Source: CAD feature listing. Evaluate the final solid. Frame: model axes, mm. A direction names the side the tool comes from. Round coordinates to 2 decimals unless told otherwise and drop trailing zeros. Order: outer loops, then holes, each group sorted by start corner. A loop starts at its lowest first (then second) coordinate and runs counter-clockwise, first axis right, second up. Notation, with made-up numbers: (11.5, 50.25) -> (47.5, 50.25) arc R29 ccw to (47.5, 85.25) -> close; hole circle Ø7 at (-26, 66). An arc over 180 degrees is marked (long way). Write item = value, one per line. Start each with the question number.
(1) Cut plane D-D on x = -1.5. Return the cut outline in (y, z), then the cut area to 3 significant figures.
(2) Draft query along Y for faces 1 (the face through (0, 11.43, 11)), 2 (the face through (0, 1, 5)), 3 (the face through (2.57, 8.7, 11.45)), 4 (the face through (-2, 0, 8)). Return one class per face: released by +Y, released by -Y, zero draft, split by the parting line, or undercut.
(3) Ray query, line 1 (X direction, y = 2, z = 5); line 2 (Z direction, x = 7.5, y = 4.25); line 3 (Z direction, x = -6.25, y = 1.5). Return the intervals inside material, ascending.
(4) Reachability of faces 5 (the face through (-5, 1, 0)), 6 (the face through (-7.5, 2.54, 5)) from +Z, -Z, +X, -X, +Y, -Y: full face, straight path, thin tool, end or side. Return the list, or none.
(5) Cut plane C-C on x = -6.25. Return the cut outline in (y, z).
(6) Cut plane B-B on z = 5.08. Return the cut outline in (x, y) (3 decimals).
(7) Cut plane A-A on y = 1.75. Return the cut outline in (x, z) (3 decimals).
(8) Contact query for flat-ended pins moving along their axis: pin 1 Ø1.3 at (y, z) = (0.5, 5) entering from +X; pin 2 Ø2.5 at (x, z) = (-5, 3) entering from +Y; pin 3 Ø6 at (y, z) = (8.5, 3) entering from +X. Output: stop coordinate, or through.
from build123d import *

# Parameters (mm, degrees)
SKETCH1_W           = 8.89
SKETCH1_H           = 12.7
SKETCH1_R           = 2.54
BOSS_EXTRUDE1_DEPTH = 2.54
SKETCH2_W           = 17.78
SKETCH2_H           = 11.43
SKETCH2_R           = 2.54
BOSS_EXTRUDE2_DEPTH = 2.54


with BuildPart() as part:
    # Sketch1 → Boss-Extrude1 (new body)
    with BuildSketch(Plane(origin=(0, 0, 0), x_dir=(1, 0, 0), z_dir=(0, 1, 0))):
        with Locations((-4.445, -6.35)):
            Rectangle(SKETCH1_W, SKETCH1_H)
        with Locations((-4.445, -5.08)):
            Circle(SKETCH1_R, mode=Mode.SUBTRACT)
    extrude(amount=BOSS_EXTRUDE1_DEPTH)

    # Sketch2 → Boss-Extrude2 (add)
    with BuildSketch(Plane.XY.offset(12.7)):
        with Locations((0, 5.715)):
            Rectangle(SKETCH2_W, SKETCH2_H)
        with Locations((4.445, 6.985)):
            Circle(SKETCH2_R, mode=Mode.SUBTRACT)
    extrude(amount=-BOSS_EXTRUDE2_DEPTH)


solid = part.part
Evaluation:
q1.outline = (0, 0) -> (2.54, 0) -> (2.54, 10.16) -> (11.43, 10.16) -> (11.43, 12.7) -> (0, 12.7) -> close
q1.area = 54.8 mm^2
q2.face_1 = released by +Y
q2.face_2 = zero draft
q2.face_3 = undercut
q2.face_4 = released by -Y
q3.line_1 = -8.89 to -6.98, -1.91 to 0
q3.line_2 = 10.16 to 12.7
q3.line_3 = 0 to 3.29, 6.87 to 12.7
q4.face_5 = -Z, +X, -X, +Y, -Y
q4.face_6 = -Z, +X, -X, +Y
q5.outline = (0, 0) -> (2.54, 0) -> (2.54, 3.29) -> (0, 3.29) -> close; (0, 6.87) -> (2.54, 6.87) -> (2.54, 10.16) -> (11.43, 10.16) -> (11.43, 12.7) -> (0, 12.7) -> close
q6.outline = (-8.89, 0) -> (-6.985, 0) -> (-6.985, 2.54) -> (-8.89, 2.54) -> close; (-1.905, 0) -> (0, 0) -> (0, 2.54) -> (-1.905, 2.54) -> close
q7.outline = (-8.89, 0) -> (0, 0) -> (0, 10.16) -> (8.89, 10.16) -> (8.89, 12.7) -> (-8.89, 12.7) -> close; hole circle Ø5.08 at (-4.445, 5.08)
q8.pin_1 = 0
q8.pin_2 = 2.54
q8.pin_3 = through
